from build123d import *

# Parameters (mm, degrees)
F0_R          = 50.8
F0_R_2        = 47.625
F1_DEPTH      = 3.81
F1_DEPTH_BACK = 50.8
F2_R          = 50.8
F2_R_2        = 49.2125
F3_DEPTH      = 50.801
F4_SIZE2      = 1.016
F4_SIZE       = 19.05


# Not quite as in the source:
# - a fillet or chamfer that OpenCascade refuses, or shapes differently, is made with other operations: its cross-section is extruded or revolved along the edge and cut away or added


with BuildPart() as f1:
    # F0 (on Front) → F1 (new body, two sides)
    with BuildSketch(Plane.XZ) as f1_sk:
        Circle(F0_R)
        Circle(F0_R_2, mode=Mode.SUBTRACT)
    extrude(amount=-F1_DEPTH)
    extrude(f1_sk.sketch, amount=F1_DEPTH_BACK)

    # F2 (on Front) → F3 (cut, through all)
    with BuildSketch(Plane.XZ):
        Circle(F2_R)
        Circle(F2_R_2, mode=Mode.SUBTRACT)
    extrude(amount=F3_DEPTH, mode=Mode.SUBTRACT)

    # F4
    f4_edges = [f1.edges().sort_by_distance(p)[0] for p in [
        (-49.2125, -50.8, 0),
    ]]
    chamfer(f4_edges, length=F4_SIZE, length2=F4_SIZE2)

    # F5: fillet of radius 5.08 on 1 edges, made by hand

    # F5_s1 → F5_t2 (revolve, cut)
    with BuildSketch(Plane.XY):
        with BuildLine():
            ThreePointArc((48.3194667684, -48.4943730928), (48.1108173968, -49.6889287689), (47.625, -50.8))
            Line((47.625, -50.8), (48.1965, -50.8))
            Line((48.1965, -50.8), (48.3194667684, -48.4943730928))
        make_face()
    revolve(axis=Axis((0, -50.8, 0), (0, 1, 0)), mode=Mode.SUBTRACT)

    # F6 (on Right) → F7 (revolve)
    with BuildSketch(Plane.YZ):
        Polygon((76.2, 76.2), (3.81, 50.8), (0, 50.8), (0, 47.407604754), (3.81, 47.407604754), (60.2590404451, 67.3254877329), align=None)
    revolve(axis=Axis((0, 38.1, 0), (0, -1, 0)))


solid = f1.part
Model file for the job. Use its own axes, mm. A direction names the side the tool comes from. Give positions to 0.01 mm unless a question says otherwise; leave off trailing zeros.
1) Wall check: line 1 (Z direction, x = 0, y = -28) (1 decimal); line 2 (Z direction, x = 0, y = 2). Give the ranges that are in metal, low to high.
2) Pull direction Z, two halves, no side cores. Call faces 1 (the cylindrical face through (-14.24, 1.93, 45.22)), 2 (the cylindrical face through (46.94, -15.65, 14.78)), 3 (the flat face through (-27, 0, 42)), 4 (the conical face through (66.266, 61.256, -14.715)): +Z half, -Z half, draft (parallel to the pull), parting line (faces both ways), or undercut.
3) Tool access for faces 5 (the conical face through (-15.279, 13.613, 48.518)), 6 (the cylindrical face through (-37.794, -25.044, -28.979)): list every direction of +Z, -Z, +X, -X, +Y, -Y with a clear straight run to the whole face (end or side of a thin tool).
4) Flat gauge pins, fed straight in: pin 1 Ø12 at (y, z) = (19.5, -27) entering from +X; pin 2 Ø12 at (y, z) = (56.5, 33) entering from +X; pin 3 Ø3 at (y, z) = (7.5, 12.5) entering from +X. Where does each tip first touch, or does it go through?
Answer block:
1. line 1: z = -49.2 to -47.6, 47.6 to 49.2
1. line 2: z = -50.8 to -47.41, 47.41 to 50.8
2. face 1: undercut
2. face 2: parting line
2. face 3: draft
2. face 4: undercut
3. face 5: +Y
3. face 6: -Y
4. pin 1: stops at x = 53.13
4. pin 2: stops at x = 64.68
4. pin 3: stops at x = 51.22
